Geometry: final body of the model. Coordinates: model frame, mm. Coordinates: 2 decimals unless noted, no trailing zeros. Order: outer loops, then holes, each group sorted by start corner. A loop starts at its lowest first (then second) coordinate and runs counter-clockwise, first axis right, second up. Notation, with made-up numbers: (81.5, 65) -> (86.5, 65) arc R18 ccw to (86.5, 89) -> close; hole circle Ø2 at (8, -20.5). An arc over 180 degrees is marked (long way). Use CSV: the item, a comma, the result in double quotes. Start each with the question number.
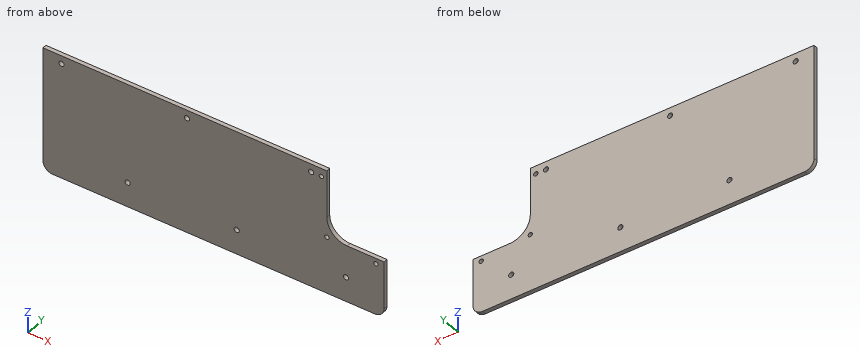
Autodesk Inventor part; units mm, degrees
ref_plane "YZ Plane" through (0, 0, 0) normal (1, 0, 0) x (0, 1, 0)
ref_plane "XZ Plane" through (0, 0, 0) normal (0, 1, 0) x (-1, 0, 0)
ref_plane "XY Plane" through (0, 0, 0) normal (0, 0, 1) x (1, 0, 0)
sketch "Sketch1" plane through (0, 0, 0) normal (0, 1, 0) x (-1, 0, 0)
  line L0 (0, 0) -> (250, 0)
  line L1 (250, 0) -> (250, -85.25)
  line L2 (243, -92.25) -> (7, -92.25)
  line L3 (0, -85.25) -> (0, 0)
  arc A0 (243, -92.25) -> (250, -85.25) centre (243, -85.25) ccw
  arc A1 (0, -85.25) -> (7, -92.25) centre (7, -85.25) ccw
  point P0 (250, -92.25)
  point P1 (0, -92.25)
  dimension "d0" = 250
  dimension "d1" = 92.25
  dimension "d2" = 7
extrude "Extrusion1" add sketch "Sketch1" along normal blind 3
sketch "Sketch2" plane through (0, 3, 0) normal (0, 1, 0) x (1, 0, 0)
  line L0 (-302.172, 6) -> (59.9962, 6) construction
  line L1 (-309.1368, 74) -> (37.3606, 74) construction
  line L2 (-7, 92.25) -> (-243, 92.25)
  line L3 (-250, 0) -> (0, 0)
  line L4 (0, 0) -> (0, 85.25)
  line L5 (-250, 85.25) -> (-250, 0)
  point P0 (-28, 74)
  point P1 (-108, 74)
  point P2 (-188, 74)
  point P3 (-53.5, 6)
  point P4 (-144.5, 6)
  point P5 (-236.5, 6)
  dimension "d5" = 18.25
  dimension "d6" = 6
  dimension "d8" = 80
  dimension "d9" = 80
  dimension "d20" = 13.5
  dimension "d22" = 196.5
  dimension "d23" = 62
  dimension "d24" = 105.5
hole "Hole1" at (-28, 3, -74) at (-108, 3, -74) at (-188, 3, -74) at (-53.5, 3, -6) at (-144.5, 3, -6) at (-236.5, 3, -6) direction (0, -1, 0) diameter 3.8 end through all
sketch "Sketch3" plane through (0, 3, 0) normal (0, 1, 0) x (1, 0, 0)
  line L0 (0, 0) -> (-42, 0)
  line L1 (-42, 0) -> (-42, 35)
  line L2 (-27, 50) -> (0, 50)
  line L3 (0, 50) -> (0, 0)
  line L4 (-250, 85.25) -> (-250, 0)
  arc A0 (-27, 50) -> (-42, 35) centre (-27, 35) ccw
  dimension "d26" = 50
  dimension "d27" = 208
  dimension "d28" = 15
extrude "Extrusion2" cut sketch "Sketch3" against normal through all
sketch "Sketch4" plane through (0, 3, 0) normal (0, 1, 0) x (1, 0, 0)
  line L0 (-46, -14.9041) -> (-46, 62.5179) construction
  line L1 (7.7091, 54) -> (-71.6012, 54) construction
  line L2 (0, 50) -> (-27, 50) construction
  line L3 (0, 50) -> (-74.4337, 50) construction
  line L4 (-250, 0) -> (-42, 0) construction
  line L5 (-42, 0) -> (-42, 52.8873) construction
  line L6 (0, 50) -> (0, 85.25)
  point P0 (0, 0)
  point P1 (-6, 54)
  point P2 (-18, 54)
  point P3 (-46, 18)
  point P4 (-46, 6)
  point P5 (-42, 50)
  dimension "d31" = 4
  dimension "d32" = 4
  dimension "d33" = 6
  dimension "d34" = 6
  dimension "d35" = 18
  dimension "d36" = 18
hole "Hole2" at (-6, 3, -54) at (-46, 3, -6) at (-42, 3, -50) direction (0, -1, 0) diameter 3.2 end through all
properties part number "Electronics cover"
(1) Section B-B (z = -12). Return loops of the section in (x, y).
(2) Section A-A (y = 1.65). State how many separate pieces and enclosed holes the cut face has, then the cut area to 3 significant figures.
(3) Line query: line 1 (X direction, y = 0.85, z = -6); line 2 (X direction, y = 1.35, z = -74); line 3 (Z direction, x = -46, y = 2.35). Output: solid intervals per line, ascending. Write a range as from..to.
(4) Section C-C (z = -38). Return loops of the section in (x, y).
(5) First-contact query: pin 1 (4 mm diameter, centred on x = -42, z = -50, fed in from -Y); pin 2 (0.9 mm diameter, centred on x = -7.5, y = 1, fed in from +Z). Flat tips, straight axial feed; report the tip coordinate or a pass-through.
Check sheet entries:
1,outline,"(-250, 0) -> (-42, 0) -> (-42, 3) -> (-250, 3) -> close"
2,separate pieces,"1"
2,enclosed holes,"9"
2,area,"20,900 mm^2"
3,line 1,"x = -250..-238.4, -234.6..-146.4, -142.6..-55.4, -51.6..-47.6, -44.4..-42"
3,line 2,"x = -250..-189.9, -186.1..-109.9, -106.1..-29.9, -26.1..0"
3,line 3,"z = -92.25..-7.6, -4.4..0"
4,outline,"(-250, 0) -> (-41.7, 0) -> (-41.7, 3) -> (-250, 3) -> close"
5,pin 1,"stops at y = 0"
5,pin 2,"stops at z = -50"
